The listing builds one solid part. Answer for the finished solid, in the listing's coordinates (mm). Round coordinates to 2 decimals unless told otherwise and drop trailing zeros. Write each loop counter-clockwise with the first axis right and the second up, starting at its lowest first coordinate (ties: lowest second). Pieces come first, ordered by that corner, then holes.
Item 1: Find the intervals of material crossed by probe 1 along Z at (x, y) = (1.2, 203.2); probe 2 along X at (y, z) = (566, 28.5) (3 decimals), in increasing order.
Item 2: Each of these flat-tipped pins is pushed along its axis until it touches: pin 1 (4 mm diameter, centred on y = 1195.5, z = 26, fed in from +X) (3 decimals); pin 2 (7.5 mm diameter, centred on x = 12.7, y = 2170.29, fed in from +Z) (3 decimals). Where does it stop, or does it pass through?
Item 3: Find section B-B on y = 2364.5. Give the vertices of the cut face in (x, z) (3 decimals), then the cut area to 3 significant figures.
Item 4: Find section A-A on z = 11. Give the vertices of the cut face in (x, y) (3 decimals).
```python
from build123d import *

# Parameters (mm, degrees)
F1_DEPTH = 2844.8
F2_R     = 3.175
F4_DEPTH = 25.4
F3_R     = 3.175
F5_DEPTH = 25.4


with BuildPart() as f1:
    # F0 (on Front) → F1 (new body)
    with BuildSketch(Plane.XZ):
        Polygon((0, 38.1), (0, 0), (38.1, 0), (38.1, 3.175), (3.175, 3.175), (3.175, 38.1), align=None)
    extrude(amount=-F1_DEPTH)

    # F2 (on Top) → F4 (cut)
    with BuildSketch(Plane.XY):
        with Locations((12.7, 76.2)):
            Circle(F2_R)
        with Locations((12.7, 375.355556)):
            Circle(F2_R)
        with Locations((12.7, 674.511111)):
            Circle(F2_R)
        with Locations((12.7, 973.666667)):
            Circle(F2_R)
        with Locations((12.7, 1272.822222)):
            Circle(F2_R)
        with Locations((12.7, 1571.977778)):
            Circle(F2_R)
        with Locations((12.7, 1871.133333)):
            Circle(F2_R)
        with Locations((12.7, 2170.288889)):
            Circle(F2_R)
        with Locations((12.7, 2469.444444)):
            Circle(F2_R)
        with Locations((12.7, 2768.6)):
            Circle(F2_R)
    extrude(amount=F4_DEPTH, mode=Mode.SUBTRACT)

    # F3 (on Right) → F5 (cut)
    with BuildSketch(Plane.YZ):
        with Locations((203.2, 20.305524)):
            Circle(F3_R)
        with Locations((508, 20.305524)):
            Circle(F3_R)
        with Locations((812.8, 20.305524)):
            Circle(F3_R)
        with Locations((1117.6, 20.305524)):
            Circle(F3_R)
        with Locations((1422.4, 20.305524)):
            Circle(F3_R)
        with Locations((1727.2, 20.305524)):
            Circle(F3_R)
        with Locations((2032, 20.305524)):
            Circle(F3_R)
        with Locations((2336.8, 20.305524)):
            Circle(F3_R)
        with Locations((2641.6, 20.305524)):
            Circle(F3_R)
    extrude(amount=F5_DEPTH, mode=Mode.SUBTRACT)


solid = f1.part
```
Check values:
1. probe 1: z = 0 to 17.13, 23.48 to 38.1
1. probe 2: x = 0 to 3.175
2. pin 1: stops at x = 3.175
2. pin 2: stops at z = 3.175
3. outline: (0, 0) - (38.1, 0) - (38.1, 3.175) - (3.175, 3.175) - (3.175, 38.1) - (0, 38.1) - close
3. area: 232 mm2
4. outline: (0, 0) - (3.175, 0) - (3.175, 2844.8) - (0, 2844.8) - close
